Design review of the part built by this model. Coordinates are the model's own, in mm. Face numbers are marked on the shaded views. A direction names the side the tool comes from. Coordinates: 2 decimals unless noted, no trailing zeros. Order: outer loops, then holes, each group sorted by start corner. A loop starts at its lowest first (then second) coordinate and runs counter-clockwise, first axis right, second up. Notation, with made-up numbers: M 61.5,-28 L 92.5,-28 A10 cw 92.5,-10 Z; hole C 79.5,62.25 d9. An arc over 180 degrees is marked long. Answer in a Markdown table with one row per item.
from build123d import *

# Parameters (mm, degrees)
SKETCH_W        = 85
SKETCH_H        = 56
PAD_DEPTH       = 5
SKETCH001_W     = 65
SKETCH001_H     = 36
POCKET_DEPTH    = 5.001
SKETCH002_R     = 3
PAD001_DEPTH    = 5
SKETCH003_R     = 1
POCKET001_DEPTH = 10.001
SKETCH004_W     = 44
SKETCH004_H     = 5
PAD002_DEPTH    = 5
PAD003_DEPTH    = 40
PAD004_DEPTH    = 21
FILLET_R        = 6
FILLET001_R     = 3
SKETCH007_W     = 22.516809
SKETCH007_H     = 5
PAD005_DEPTH    = 25
FILLET002_R     = 5
FILLET003_R     = 5
SKETCH008_R     = 2.5
POCKET002_DEPTH = 5.001
SKETCH009_R     = 1.5
SKETCH009_R_2   = 2
POCKET003_DEPTH = 12.001


with BuildPart() as part:
    # Sketch → Pad (new body)
    with BuildSketch(Plane.XY):
        Rectangle(SKETCH_W, SKETCH_H)
    extrude(amount=PAD_DEPTH)

    # Sketch001 → Pocket (cut, through all)
    with BuildSketch(Plane.XY.offset(5)):
        Rectangle(SKETCH001_W, SKETCH001_H)
    extrude(amount=-POCKET_DEPTH, mode=Mode.SUBTRACT)

    # Sketch002 → Pad001 (new body)
    with BuildSketch(Plane.XY.offset(5)):
        with Locations((39, 24.5)):
            Circle(SKETCH002_R)
        with Locations((-18.5, 24.5)):
            Circle(SKETCH002_R)
        with Locations((-18.5, -24.5)):
            Circle(SKETCH002_R)
        with Locations((39, -24.5)):
            Circle(SKETCH002_R)
    extrude(amount=PAD001_DEPTH)

    # Sketch003 → Pocket001 (cut, through all)
    with BuildSketch(Plane.XY.offset(10)):
        with Locations((-18.5, 24.5)):
            Circle(SKETCH003_R)
        with Locations((-18.5, -24.5)):
            Circle(SKETCH003_R)
        with Locations((39, 24.5)):
            Circle(SKETCH003_R)
        with Locations((39, -24.5)):
            Circle(SKETCH003_R)
    extrude(amount=-POCKET001_DEPTH, mode=Mode.SUBTRACT)

    # Sketch004 → Pad002 (new body)
    with BuildSketch(Plane.YZ.offset(42.5)):
        with Locations((-6, 2.5)):
            Rectangle(SKETCH004_W, SKETCH004_H)
    extrude(amount=PAD002_DEPTH)

    # Sketch005 → Pad003 (new body)
    with BuildSketch(Plane(origin=(0, 0, 0), x_dir=(1, 0, 0), z_dir=(0, 0, -1))):
        Polygon((45.5, 28), (45.5, 24), (47.5, 24), (47.5, 26), (58.5, 26), (58.5, 24), (60.5, 24), (60.5, 28), align=None)
        Polygon((45.5, -16), (45.5, -12), (47.5, -12), (47.5, -14), (58.5, -14), (58.5, -12), (60.5, -12), (60.5, -16), align=None)
    extrude(amount=-PAD003_DEPTH)

    # Sketch006 → Pad004 (new body)
    with BuildSketch(Plane(origin=(0, 16, 0), x_dir=(-1, 0, 0), z_dir=(0, 1, 0))):
        Polygon((-42.5, 0), (-42.5, 5), (-45.5, 5), (-45.5, 12), (-70.5, 12), (-70.5, 6), (-60.5, 6), (-60.5, 0), align=None)
    extrude(amount=PAD004_DEPTH)

    # Fillet
    fillet_edges = [part.edges().sort_by_distance(p)[0] for p in [
        (45.5, 26.5, 12),
    ]]
    fillet(fillet_edges, radius=FILLET_R)

    # Fillet001
    fillet001_edges = [part.edges().sort_by_distance(p)[0] for p in [
        (42.5, 37, 2.5),
    ]]
    fillet(fillet001_edges, radius=FILLET001_R)

    # Sketch007 → Pad005 (new body)
    with BuildSketch(Plane.XZ.offset(28)):
        with Locations((-15.882882, 2.5)):
            Rectangle(SKETCH007_W, SKETCH007_H)
    extrude(amount=PAD005_DEPTH)

    # Fillet002
    fillet002_edges = [part.edges().sort_by_distance(p)[0] for p in [
        (32.5, 18, 2.5),
        (32.5, -18, 2.5),
        (-32.5, -18, 2.5),
        (-42.5, 28, 2.5),
        (-42.5, -28, 2.5),
        (-27.141287, -28, 2.5),
        (-27.141287, -53, 2.5),
        (-4.624478, -53, 2.5),
        (-4.624478, -28, 2.5),
        (-32.5, 18, 2.5),
    ]]
    fillet(fillet002_edges, radius=FILLET002_R)

    # Fillet003
    fillet003_edges = [part.edges().sort_by_distance(p)[0] for p in [
        (42.5, 28, 2.5),
    ]]
    fillet(fillet003_edges, radius=FILLET003_R)

    # Sketch008 → Pocket002 (cut, through all)
    with BuildSketch(Plane.XY.offset(5)):
        with Locations((-14.5, -42)):
            Circle(SKETCH008_R)
    extrude(amount=-POCKET002_DEPTH, mode=Mode.SUBTRACT)

    # Sketch009 → Pocket003 (cut, through all)
    with BuildSketch(Plane.XY.offset(12)):
        with Locations((64.5, 31)):
            Circle(SKETCH009_R)
        with Locations((64.5, 21)):
            Circle(SKETCH009_R_2)
    extrude(amount=-POCKET003_DEPTH, mode=Mode.SUBTRACT)


solid = part.part
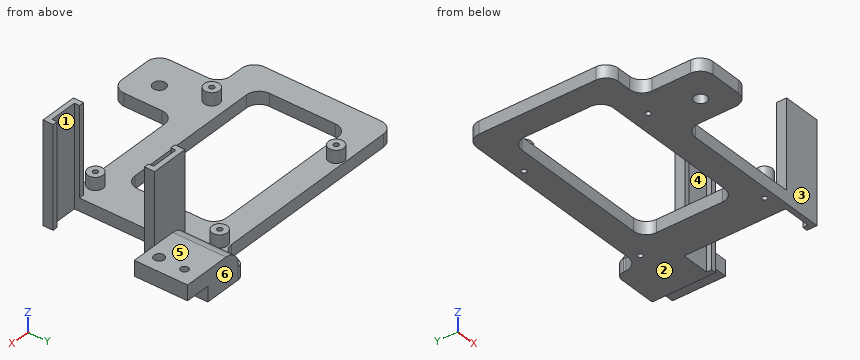
(1) Add section C-C, the plane z = 38. Give the boundary of the cut face in (x, y), and give its area (3 significant figures).
Return value:
| item | result |
|---|---|
| outline | M 45.5,-28 L 60.5,-28 L 60.5,-24 L 58.5,-24 L 58.5,-26 L 47.5,-26 L 47.5,-24 L 45.5,-24 Z; M 45.5,12 L 47.5,12 L 47.5,14 L 58.5,14 L 58.5,12 L 60.5,12 L 60.5,16 L 45.5,16 Z |
| area | 76.0 mm2 |
(2) For line 1 along Y through (x, z) = (39, 6); line 2 along X through (y, z) = (7.5, 2.5); line 3 along Y through (x, z) = (64.5, 8.05), list the stretches that pass through material, from the lowest coordinate up. Write a range as from..to.
Return value:
| item | result |
|---|---|
| line 1 | y = -27.5..-25.5, -23.5..-21.5, 21.5..23.5, 25.5..27.5 |
| line 2 | x = -42.5..-32.5, 32.5..47.5 |
| line 3 | y = 16..19, 23..29.5, 32.5..37 |
(3) Add section D-D, the plane x = 64.5. Give the boundary of the cut face in (y, z), and give its area (3 significant figures).
Return value:
| item | result |
|---|---|
| outline | M 16,6 L 19,6 L 19,12 L 16,12 Z; M 23,6 L 29.5,6 L 29.5,12 L 23,12 Z; M 32.5,6 L 37,6 L 37,12 L 32.5,12 Z |
| area | 84.0 mm2 |
(4) Add section B-B, the plane y = -42. Give the boundary of the cut face in (x, z).
Return value:
| item | result |
|---|---|
| outline | M -27.14,0 L -17,0 L -17,5 L -27.14,5 Z; M -12,0 L -4.62,0 L -4.62,5 L -12,5 Z |
(5) Add section A-A, the plane x = 7.5. Give the boundary of the cut face in (y, z), and give its area (3 significant figures).
Return value:
| item | result |
|---|---|
| outline | M -28,0 L -18,0 L -18,5 L -28,5 Z; M 18,0 L 28,0 L 28,5 L 18,5 Z |
| area | 100 mm2 |
(6) For the marked faces 4, 5 and 6, list the 3-axis set-ups (+Z, -Z, +X, -X, +Y, -Y) from which the entire face can be reached by the end or side of a thin tool; tool diameter is ignored.
Return value:
| item | result |
|---|---|
| face 4 | +Z, -Z |
| face 5 | +Z, +X, -X, +Y |
| face 6 | +Z, -Z, +X, -X, +Y |
(7) Draft analysis for pull direction Y (two halves, no side actions). For the marked faces 1, 2 and 3, state which applies: pulls with the +Y half, pulls with the -Y half, needs draft (parallel to the pull), parting line crosses it, or undercut.
Return value:
| item | result |
|---|---|
| face 1 | undercut |
| face 2 | needs draft |
| face 3 | pulls with the -Y half |
(8) Insertion check: pin 1 Ø2 at (y, z) = (-25, 13) entering from +X; pin 2 Ø6.5 at (x, y) = (-18, -23.5) entering from +Z; pin 3 Ø4.5 at (x, y) = (64.5, 21) entering from -Z; pin 4 Ø4 at (x, y) = (-14.5, -42) entering from -Z. Each pin has a flat end and moves straight along its axis. Give the tip position at first contact, or say it passes through.
Return value:
| item | result |
|---|---|
| pin 1 | stops at x = 60.5 |
| pin 2 | stops at z = 10 |
| pin 3 | stops at z = 6 |
| pin 4 | passes through |
